from build123d import *

# Parameters (mm, degrees)
F0_R     = 2.75
F0_R_2   = 3
F1_DEPTH = 9.9
F2_DEPTH = 7.9
F3_R     = 8
F3_R_2   = 3
F4_DEPTH = 5
F5_R     = 2
F6_SIZE  = 0.5


with BuildPart() as f1:
    # F0 (on Top) → F1 (new body)
    with BuildSketch(Plane.XY):
        Polygon((-9.7113248654, -16.8205080757), (0, -33.6410161514), (9.7113248654, -16.8205080757), align=None)
        with Locations((0, -23.0940107676)):
            Circle(F0_R, mode=Mode.SUBTRACT)
        Polygon((-19.4226497308, 0), (-9.7113248654, -16.8205080757), (9.7113248654, -16.8205080757), (19.4226497308, 0), (9.7113248654, 16.8205080757), (-9.7113248654, 16.8205080757), align=None)
        Circle(F0_R_2, mode=Mode.SUBTRACT)
        Polygon((-29.1339745962, 16.8205080757), (-19.4226497308, 0), (-9.7113248654, 16.8205080757), align=None)
        with Locations((-20, 11.5470053838)):
            Circle(F0_R, mode=Mode.SUBTRACT)
        Polygon((9.7113248654, 16.8205080757), (19.4226497308, 0), (29.1339745962, 16.8205080757), align=None)
        with Locations((20, 11.5470053838)):
            Circle(F0_R, mode=Mode.SUBTRACT)
    extrude(amount=F1_DEPTH)

    # F0 (on Top) → F2 (cut)
    with BuildSketch(Plane.XY):
        Polygon((9.7113248654, 16.8205080757), (19.4226497308, 0), (29.1339745962, 16.8205080757), align=None)
        with Locations((20, 11.5470053838)):
            Circle(F0_R, mode=Mode.SUBTRACT)
        Polygon((-9.7113248654, -16.8205080757), (0, -33.6410161514), (9.7113248654, -16.8205080757), align=None)
        with Locations((0, -23.0940107676)):
            Circle(F0_R, mode=Mode.SUBTRACT)
        Polygon((-29.1339745962, 16.8205080757), (-19.4226497308, 0), (-9.7113248654, 16.8205080757), align=None)
        with Locations((-20, 11.5470053838)):
            Circle(F0_R, mode=Mode.SUBTRACT)
    extrude(amount=F2_DEPTH, mode=Mode.SUBTRACT)

    # F3 (on face) → F4 (cut)
    with BuildSketch(Plane.XY.offset(9.9)):
        Circle(F3_R)
        Circle(F3_R_2, mode=Mode.SUBTRACT)
    extrude(amount=-F4_DEPTH, mode=Mode.SUBTRACT)

    # F5
    f5_edges = [f1.edges().sort_by_distance(p)[0] for p in [
        (-29.133975, 16.820508, 8.9),
        (-9.711325, 16.820508, 3.95),
        (-19.42265, 0, 3.95),
        (9.711325, 16.820508, 3.95),
        (14.566987, 8.410254, 0),
        (0, 16.820508, 0),
        (-14.566987, 8.410254, 0),
        (-14.566987, -8.410254, 0),
        (0, -16.820508, 0),
        (19.42265, 0, 3.95),
        (9.711325, -16.820508, 3.95),
        (0, -33.641016, 8.9),
        (29.133975, 16.820508, 8.9),
        (-9.711325, -16.820508, 3.95),
        (14.566987, -8.410254, 0),
    ]]
    fillet(f5_edges, radius=F5_R)

    # F6
    f6_edges = [f1.edges().sort_by_distance(p)[0] for p in [
        (0, -31.641016, 7.9),
        (-27.401924, 15.820508, 7.9),
        (27.401924, 15.820508, 7.9),
    ]]
    chamfer(f6_edges, length=F6_SIZE)


solid = f1.part
Geometry: final body of the model. Coordinates: model frame, mm. A direction names the side the tool comes from. Give positions to 0.01 mm unless a question says otherwise; leave off trailing zeros. Loops run counter-clockwise (first coordinate to the right, second up) from the corner with the lowest first, then second, coordinate; pieces in that order, holes last. Notation, with made-up numbers: M 80,81 L 115,81 A18 ccw 115,106 Z; hole C 15.5,74 d7. An arc over 180 degrees is marked long. Put each result on its own line as item: value. Start each with the question number.
1) Cut plane A-A (x = 20). Output: boundary loops of the cut face in (y, z), then the cut area to 3 significant figures.
2) Contact query for flat-ended pins moving along their axis: pin 1 (8 mm diameter, centred on x = -22.5, y = 6.5, fed in from -Z); pin 2 (4 mm diameter, centred on y = 3, z = 8.5, fed in from -X); pin 3 (4 mm diameter, centred on x = 0, z = 6, fed in from -Y); pin 4 (3.5 mm diameter, centred on x = -20, y = 11.55, fed in from -Z). Output: stop coordinate, or through.
3) Cut plane C-C (x = -6.5). Output: boundary loops of the cut face in (y, z).
4) Access query for faces 4 (the flat face through (-14.627, 8.307, 4.909)), 5 (the cylindrical face through (19.113, -0.015, 5.245)), 6 (the flat face through (14.51, 8.51, 4.91)), 7 (the flat face through (0, -16.821, 5)), 8 (the cylindrical face through (-9.54, -16.56, 5.24)). Directions: +Z, -Z, +X, -X, +Y, -Y. A direction counts if a zero-diameter tool reaches every point of the face in a straight line with its end or side. Return the directions, or none.
5) Ray query, line 1 along Y through (x, z) = (0, 3.55); line 2 along Z through (x, y) = (4, -22); line 3 along X through (y, z) = (-1.5, 9). Return the intervals inside material, ascending.
6) Cut plane B-B (x = 0). Output: boundary loops of the cut face in (y, z).
7) Pull-direction query (Y, two-part tool) for faces 1 (the cylindrical face through (14.106, 8.006, 0.57)), 2 (the cylindrical face through (-22.747, 11.668, 8.886)), 3 (the flat face through (-14.747, -8.099, 6.772)); classes: pulls with the +Y half, pulls with the -Y half, needs draft (parallel to the pull), parting line crosses it, or undercut.
Verdict:
1. outline: M 1,8.4 L 2,7.9 L 8.8,7.9 L 8.8,9.9 L 1,9.9 Z; M 14.3,7.9 L 16.32,7.9 L 16.82,8.4 L 16.82,9.9 L 14.3,9.9 Z
1. area: 20.3 mm2
2. pin 1: z = 7.9
2. pin 2: x = -22.31
2. pin 3: y = -31.24
2. pin 4: through
3. outline: M -22.38,8.4 L -21.38,7.9 L -16.82,7.9 L -16.82,2 A2 ccw -14.82,0 L 14.82,0 A2 ccw 16.82,2 L 16.82,9.9 L 4.66,9.9 L 4.66,4.9 L -4.66,4.9 L -4.66,9.9 L -22.38,9.9 Z
4. face 4: -Z, -X, +Y
4. face 5: -Z, +X
4. face 6: -Z, +X, +Y
4. face 7: -Z, +X, -X, -Y
4. face 8: -Z, -X, -Y
5. line 1: -16.82 to -3, 3 to 16.82
5. line 2: 7.9 to 9.9
5. line 3: -18.56 to -7.86, 7.86 to 18.56
6. outline: M -31.64,8.4 L -31.14,7.9 L -25.84,7.9 L -25.84,9.9 L -31.64,9.9 Z; M -20.34,7.9 L -16.82,7.9 L -16.82,2 A2 ccw -14.82,0 L -3,0 L -3,4.9 L -8,4.9 L -8,9.9 L -20.34,9.9 Z; M 3,0 L 14.82,0 A2 ccw 16.82,2 L 16.82,9.9 L 8,9.9 L 8,4.9 L 3,4.9 Z
7. face 1: pulls with the +Y half
7. face 2: undercut
7. face 3: pulls with the -Y half
